Read the model definition and answer for the solid it produces. Units are mm, in the model's axes. A direction names the side the tool comes from. Give positions to 0.01 mm unless a question says otherwise; leave off trailing zeros. Order: outer loops, then holes, each group sorted by start corner. A loop starts at its lowest first (then second) coordinate and runs counter-clockwise, first axis right, second up. Notation, with made-up numbers: (-21, -27.75) - (-3, -27.75) arc R14 ccw to (-3, -14.75) - close; hole circle Ø8 at (35.5, 1). An arc over 180 degrees is marked (long way). Return JSON: item names as keys, results as strings.
```python
from build123d import *

# Parameters (mm, degrees)
SKETCH1_W            = 500
SKETCH1_H            = 400
BOSS_EXTRUDE1_DEPTH  = 12
SKETCH2_W            = 12
SKETCH2_H            = 133.333333333
CUT_EXTRUDE1_DEPTH   = 12
SCALE1_SCALE         = 0.5
M3_CLEARANCE_SLOT1_D = 3.4


with BuildPart() as part:
    # Sketch1 → Boss-Extrude1 (new body)
    with BuildSketch(Plane.XY):
        with Locations((250, 200)):
            Rectangle(SKETCH1_W, SKETCH1_H)
    extrude(amount=BOSS_EXTRUDE1_DEPTH)

    # Sketch2 → Cut-Extrude1 (cut)
    with BuildSketch(Plane.XY.offset(12)):
        with Locations((494, 333.333333334)):
            Rectangle(SKETCH2_W, SKETCH2_H)
        with Locations((6, 333.333333334)):
            Rectangle(SKETCH2_W, SKETCH2_H)
        with Locations((6, 66.666666667)):
            Rectangle(SKETCH2_W, SKETCH2_H)
        with Locations((494, 66.666666667)):
            Rectangle(SKETCH2_W, SKETCH2_H)
    extrude(amount=-CUT_EXTRUDE1_DEPTH, mode=Mode.SUBTRACT)


with BuildPart() as part_1:
    # Scale1: scaled about (250, 200, 6)
    add(part.part.scale(SCALE1_SCALE).moved(Location((125, 100, 3))))

    # M3 Clearance Slot1 (through all)
    with Locations(Plane(origin=(0, 0, 3), x_dir=(-1, 0, 0), z_dir=(0, 0, -1))):
        with Locations((-372, 211.113333333), (-372, 188.886666667), (-128, 211.11), (-128, 188.89)):
            Hole(M3_CLEARANCE_SLOT1_D / 2)


solid = part_1.part
```
Q1. A cutting plane is placed at A-A (z = 7). Write down the section's boundary in (x, y).
Values:
{"outline": "(125, 166.67) - (131, 166.67) - (131, 100) - (369, 100) - (369, 166.67) - (375, 166.67) - (375, 233.33) - (369, 233.33) - (369, 300) - (131, 300) - (131, 233.33) - (125, 233.33) - close; hole circle Ø3.4 at (128, 188.89); hole circle Ø3.4 at (128, 211.11); hole circle Ø3.4 at (372, 188.89); hole circle Ø3.4 at (372, 211.11)"}
Q2. Consider L1, parallel to Y at x = 128, z = 7.4; L2, parallel to X at y = 188.89, z = 6.9; L3, parallel to X at y = 269, z = 5.25. Determine where each line is inside the solid, lowest interval first.
Values:
{"L1": "y = 166.67 to 187.19, 190.59 to 209.41, 212.81 to 233.33", "L2": "x = 125 to 126.3, 129.7 to 370.3, 373.7 to 375", "L3": "x = 131 to 369"}
Q3. Given pin 1 (1.8 mm diameter, centred on y = 128, z = 7.5, fed in from -X); pin 2 (3 mm diameter, centred on y = 252, z = 5.5, fed in from +X); pin 3 (1.8 mm diameter, centred on x = 372.5, z = 7, fed in from +Y), each flat-ended and moving along its own axis, determine where each tip first touches the part or whether it passes through.
Values:
{"pin 1": "stops at x = 131", "pin 2": "stops at x = 369", "pin 3": "stops at y = 233.33"}
Q4. Determine the mould class of faces 4 (the flat face through (248, 201, 3)), 5 (the flat face through (369, 266, 6)), 6 (the flat face through (125, 200, 6)) for opening direction X: released by +X, released by -X, zero draft, split by the parting line, or undercut.
Values:
{"face 4": "zero draft", "face 5": "released by +X", "face 6": "released by -X"}
Q5. For faces 1 (the flat face through (372, 166.667, 6)), 2 (the flat face through (128, 233.333, 6)), 3 (the flat face through (372, 233.333, 6)), determine the directions among +Z, -Z, +X, -X, +Y, -Y from which every point of the face is accessible in a straight line to the end or side of a thin tool.
Values:
{"face 1": "+Z, -Z, +X, -Y", "face 2": "+Z, -Z, -X, +Y", "face 3": "+Z, -Z, +X, +Y"}
Q6. A cutting plane is placed at B-B (y = 258). Write down the section's boundary in (x, z).
Values:
{"outline": "(131, 3) - (369, 3) - (369, 9) - (131, 9) - close"}
